Design review of the part shown in the three views and the two pictorial views. Dimensions are in mm from the part's minimum x, y and z. A direction names the side the tool comes from. Coordinates: 2 decimals unless noted, no trailing zeros. Loops run counter-clockwise (first coordinate to the right, second up) from the corner with the lowest first, then second, coordinate; pieces in that order, holes last.
Q1. Add section D-D on x = 13.75. Give the boundary of the cut face in (y, z), and give its area (3 significant figures).
Q2. Machinability: for the marked faces 1 and 2, which of the approach directions +Z, -Z, +X, -X, +Y, -Y give a long, thin tool a straight path to every point of the face, cutting with its end or side? Answer none if there is none.
Q3. Add section C-C on z = 1.85. Give the boundary of the cut face in (x, y), and give its area (3 significant figures).
Q4. Draft analysis for pull direction Y (two halves, no side actions). For the marked faces 3, 4 and 5, state which applies: released by +Y, released by -Y, zero draft, split by the parting line, or undercut.
Q5. For P1, Ø1, axis at y = 6, z = 1, coming from the -X side; P2, Ø1.5, axis at x = 12, z = 1, coming from the +Y side, all flat-tipped, find the tip position at first contact; note any pin that passes through.
Q6. Wall thickness on probe 1 along Y at (x, z) = (4, 1.35); probe 2 along X at (y, z) = (9.5, 2.6); probe 3 along X at (y, z) = (6.75, 1.25): over which ranges is each line inside the solid? List them lowest first.
Q7. Add section B-B on x = 4. Give the boundary of the cut face in (y, z).
Q8. Add section A-A on y = 10.75. Give the boundary of the cut face in (x, z), and give its area (3 significant figures).
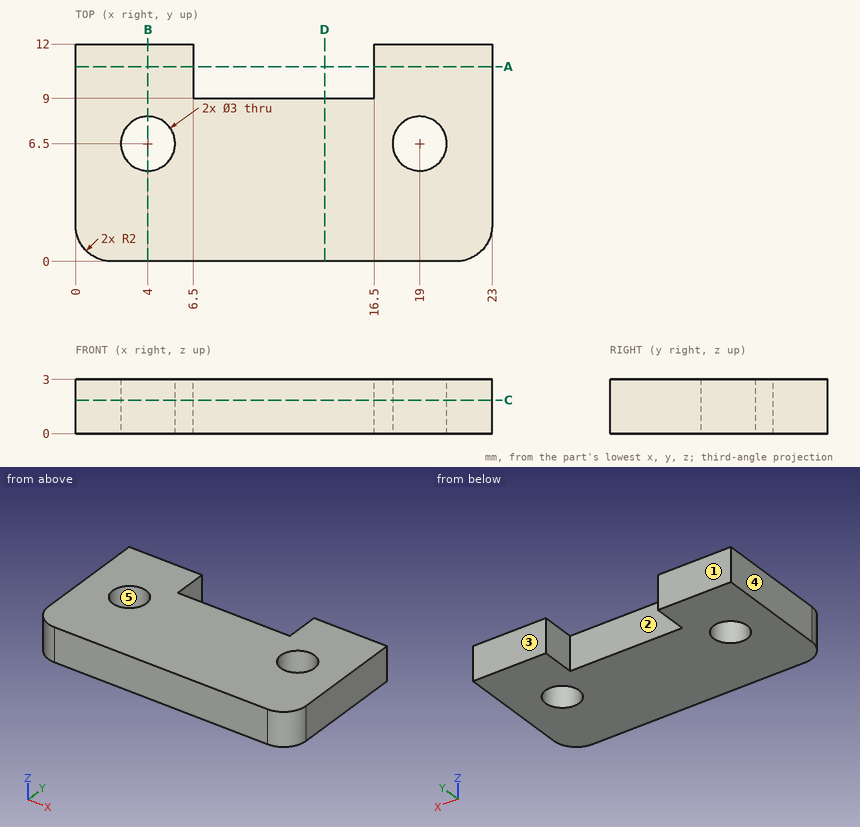
Entries:
1. outline: (0, 0) - (9, 0) - (9, 3) - (0, 3) - close
1. area: 27.0 mm2
2. face 1: +Z, -Z, +X, -X, +Y
2. face 2: +Z, -Z, +Y
3. outline: (0, 2) arc R2 ccw to (2, 0) - (21, 0) arc R2 ccw to (23, 2) - (23, 12) - (16.5, 12) - (16.5, 9) - (6.5, 9) - (6.5, 12) - (0, 12) - close; hole circle Ø3 at (4, 6.5); hole circle Ø3 at (19, 6.5)
3. area: 230 mm2
4. face 3: released by +Y
4. face 4: zero draft
4. face 5: undercut
5. P1: stops at x = 0
5. P2: stops at y = 9
6. probe 1: y = 0 to 5, 8 to 12
6. probe 2: x = 0 to 6.5, 16.5 to 23
6. probe 3: x = 0 to 2.52, 5.48 to 17.52, 20.48 to 23
7. outline: (0, 0) - (5, 0) - (5, 3) - (0, 3) - close; (8, 0) - (12, 0) - (12, 3) - (8, 3) - close
8. outline: (0, 0) - (6.5, 0) - (6.5, 3) - (0, 3) - close; (16.5, 0) - (23, 0) - (23, 3) - (16.5, 3) - close
8. area: 39.0 mm2
